The listing builds one solid part. Answer for the finished solid, in the listing's coordinates (mm). Coordinates: 2 decimals unless noted, no trailing zeros. Order: outer loops, then holes, each group sorted by start corner. A loop starts at its lowest first (then second) coordinate and runs counter-clockwise, first axis right, second up. Notation, with made-up numbers: (-15, -30) - (16, -30) arc R24 cw to (16, -8) - close; hole circle Ø3 at (81, -39). An arc over 180 degrees is marked (long way). Use a Markdown table: item, result. Add a question column.
Item 1: The mould has two halves that part along X. Classify faces 1 (the flat face through (24, 0, 10)), 2 (the flat face through (2.7, 0, 5)), 3 (the cylindrical face through (-3.2, -0.1, 4.9)), 4 (the flat face through (38.22, 3.934, 4.93)): released by +X, released by -X, zero draft, split by the parting line, or undercut.
Item 2: The part is cut by section B-B, the plane y = 4. Give the vertices of the cut face in (x, z).
Item 3: The part is cut by section A-A, the plane z = 4. Give the vertices of the cut face in (x, y) (3 decimals).
Item 4: Flat-ended cylindrical pins translate along their axes: P1, Ø1.7, axis at y = -1, z = 5, coming from the -X side; P2, Ø5, axis at x = 53.5, y = 0.5, coming from the -Z side; P3, Ø5, axis at x = 41.5, z = 9, coming from the -Y side; P4, Ø1, axis at x = 28.5, z = 5.5, coming from the +Y side. Find the tip coordinate at first contact, or state that the pin passes through.
Item 5: Find the intervals of material crossed by line 1 along Y through (x, z) = (0, 2.5); line 2 along X through (y, z) = (0.25, 0.5); line 3 along Y through (x, z) = (57, 7.25), in increasing order.
Item 6: The part is cut by section C-C, the plane x = 5. Give the vertices of the cut face in (y, z).
from build123d import *

# Parameters (mm, degrees)
F1_DEPTH = 10
F2_R     = 0.5


with BuildPart() as f1:
    # F0 (on Top) → F1 (new body)
    with BuildSketch(Plane.XY):
        with BuildLine():
            ThreePointArc((1.3939980639, -7.3693126815), (5.7751617068, -4.7851339856), (7.5, 0))
            ThreePointArc((7.5, 0), (5.5463248947, 5.048591899), (0.7031252901, 7.4669682487))
            ThreePointArc((0.7031252901, 7.4669682487), (-7.4917375109, 0.3519503765), (0, -7.5))
            Line((0, -7.5), (1.3939980639, -7.3693126815))
        make_face()
        with BuildLine():
            ThreePointArc((2.7, -1.7175564037), (-3.2, 0), (2.7, 1.7175564037))
            Line((2.7, 1.7175564037), (2.7, 0))
            Line((2.7, 0), (2.7, -1.7175564037))
        make_face(mode=Mode.SUBTRACT)
        with BuildLine():
            ThreePointArc((0.7031252901, 7.4669682487), (5.5463248947, 5.048591899), (7.5, 0))
            Line((7.5, 0), (80, 0))
            Line((80, 0), (0.7031252901, 7.4669682487))
        make_face()
        with BuildLine():
            Line((80, 0), (7.5, 0))
            ThreePointArc((7.5, 0), (5.7751617068, -4.7851339856), (1.3939980639, -7.3693126815))
            Line((1.3939980639, -7.3693126815), (80, 0))
        make_face()
    extrude(amount=F1_DEPTH)

    # F2
    f2_edges = [f1.edges().sort_by_distance(p)[0] for p in [
        (80, 0, 5),
    ]]
    fillet(f2_edges, radius=F2_R)


solid = f1.part
Solution:
| question | item | result |
|---|---|---|
| 1 | face 1 | zero draft |
| 1 | face 2 | undercut |
| 1 | face 3 | undercut |
| 1 | face 4 | released by +X |
| 2 | outline | (-6.34, 0) - (37.52, 0) - (37.52, 10) - (-6.34, 10) - close |
| 3 | outline | (0, -7.5) - (74.702, -0.497) arc R0.5 ccw to (74.702, 0.499) - (0.703, 7.467) arc R7.5 ccw (long way) to start; hole (2.7, -1.718) - (2.7, 1.718) arc R3.2 ccw (long way) to start |
| 4 | P1 | stops at x = -7.5 |
| 4 | P2 | stops at z = 0 |
| 4 | P3 | stops at y = -3.84 |
| 4 | P4 | stops at y = 4.9 |
| 5 | line 1 | y = -7.5 to -3.2, 3.2 to 7.5 |
| 5 | line 2 | x = -7.5 to -3.19, 2.7 to 75.09 |
| 5 | line 3 | y = -2.16 to 2.17 |
| 6 | outline | (-7.03, 0) - (7.06, 0) - (7.06, 10) - (-7.03, 10) - close |
